Read the model definition and answer for the solid it produces. Units are mm, in the model's axes. A direction names the side the tool comes from. Give positions to 0.01 mm unless a question says otherwise; leave off trailing zeros. Loops run counter-clockwise (first coordinate to the right, second up) from the corner with the lowest first, then second, coordinate; pieces in that order, holes last. Notation, with made-up numbers: (35, -10) -> (66, -10) arc R30 ccw to (66, 13) -> close; hole circle Ø6 at (40, -6.75). An arc over 180 degrees is marked (long way). Return JSON: item names as keys, results as strings. Group by question number.
from build123d import *

# Parameters (mm, degrees)
SKETCH2_R           = 1.7
SKETCH2_R_2         = 2.5527
SKETCH2_R_3         = 1
SKETCH2_R_4         = 6.275
BOSS_EXTRUDE1_DEPTH = 5.588
FILLET1_R           = 6.35
FILLET2_R           = 3.175


with BuildPart() as part:
    # Sketch2 → Boss-Extrude1 (new body)
    with BuildSketch(Plane.XY):
        Polygon((-44.45, 12.7), (-101.6, 12.7), (-101.6, 6.35), (-107.95, 6.35), (-107.95, 3.175), (-101.6, 3.175), (-101.6, -3.175), (-107.95, -3.175), (-107.95, -6.35), (-101.6, -6.35), (-101.6, -12.7), (85.725, -12.7), (85.725, -20.9775), (92.075, -20.9775), (92.075, -12.7), (101.6, -12.7), (101.6, 12.7), (92.075, 12.7), (92.075, 20.9775), (85.725, 20.9775), (85.725, 12.7), (44.45, 12.7), (44.45, 15.875), (41.275, 15.875), (41.275, 12.7), (34.925, 12.7), (34.925, 15.875), (31.75, 15.875), (31.75, 12.7), (-31.75, 12.7), (-31.75, 15.875), (-34.925, 15.875), (-34.925, 12.7), (-41.275, 12.7), (-41.275, 15.875), (-44.45, 15.875), align=None)
        with BuildLine():
            ThreePointArc((-92.075, -3.175), (-95.25, 0), (-92.075, 3.175))
            Line((-92.075, 3.175), (-73.025, 3.175))
            ThreePointArc((-73.025, 3.175), (-69.85, 0), (-73.025, -3.175))
            Line((-73.025, -3.175), (-92.075, -3.175))
        make_face(mode=Mode.SUBTRACT)
        with Locations((-53.975, -9.525)):
            Circle(SKETCH2_R, mode=Mode.SUBTRACT)
        with Locations((-38.1, 0)):
            Circle(SKETCH2_R_2, mode=Mode.SUBTRACT)
        with Locations((-12.7, 0)):
            Circle(SKETCH2_R_2, mode=Mode.SUBTRACT)
        with Locations((88.9, -16.215)):
            Circle(SKETCH2_R_3, mode=Mode.SUBTRACT)
        with Locations((12.7, 0)):
            Circle(SKETCH2_R_2, mode=Mode.SUBTRACT)
        with Locations((38.1, 0)):
            Circle(SKETCH2_R_2, mode=Mode.SUBTRACT)
        with Locations((69.85, -9.525)):
            Circle(SKETCH2_R, mode=Mode.SUBTRACT)
        with Locations((88.9, 0)):
            Circle(SKETCH2_R_4, mode=Mode.SUBTRACT)
        with Locations((-53.975, 9.525)):
            Circle(SKETCH2_R, mode=Mode.SUBTRACT)
        with Locations((69.85, 9.525)):
            Circle(SKETCH2_R, mode=Mode.SUBTRACT)
        with Locations((88.9, 16.215)):
            Circle(SKETCH2_R_3, mode=Mode.SUBTRACT)
    extrude(amount=BOSS_EXTRUDE1_DEPTH)

    # Fillet1
    fillet1_edges = [part.edges().sort_by_distance(p)[0] for p in [
        (101.6, -12.7, 2.794),
        (101.6, 12.7, 2.794),
        (-101.6, -12.7, 2.794),
        (-101.6, 12.7, 2.794),
        (85.725, -12.7, 2.794),
        (85.725, 12.7, 2.794),
    ]]
    fillet(fillet1_edges, radius=FILLET1_R - 0.0001)  # a hair under: the kernel refuses the full size

    # Fillet2
    fillet2_edges = [part.edges().sort_by_distance(p)[0] for p in [
        (85.725, -20.9775, 2.794),
        (92.075, -20.9775, 2.794),
        (92.075, -12.7, 2.794),
        (92.075, 12.7, 2.794),
        (92.075, 20.9775, 2.794),
        (85.725, 20.9775, 2.794),
    ]]
    fillet(fillet2_edges, radius=FILLET2_R)


solid = part.part
1. Section B-B on z = 4.4 is taken. State how many separate pieces and enclosed holes the cut face has, then the cut area to 3 significant figures.
2. Straight lines are drawn through the part: line 1 (Y direction, x = 88.9, z = 3.7) (1 decimal); line 2 (Y direction, x = -77, z = 4.5) (3 decimals); line 3 (X direction, y = -8, z = 3.6). For each, find the intervals that lie inside material, in ascending order. Write a range as from..to.
3. Determine the mould class of faces 6 (the flat face through (-69, 12.7, 3)), 7 (the flat face through (-38, 12.7, 3)), 8 (the cylindrical face through (99.69, -10.89, 2.83)) for opening direction X: pulls with the +X half, pulls with the -X half, needs draft (parallel to the pull), parting line crosses it, or undercut.
4. Section A-A on x = -12.7 is taken. Determine the outline of the cut face in (y, z), then the cut area to 3 significant figures.
5. Which of the six approach directions +Z, -Z, +X, -X, +Y, -Y give full straight-line access (tool end or side, diameter ignored) to faces 1 (the flat face through (-105, -3.175, 3)), 2 (the flat face through (-9, -12.7, 3)), 3 (the flat face through (-105, 6.35, 3)), 4 (the flat face through (38, 12.7, 3)), 5 (the flat face through (-83, 3.175, 3))?
6. Flat-ended cylindrical pins translate along their axes: pin 1 Ø3 at (y, z) = (1, 3) entering from -X; pin 2 Ø3 at (x, z) = (-106, 1.5) entering from +Y; pin 3 Ø2.5 at (x, z) = (-43.5, 2.5) entering from +Y (3 decimals). Find the tip coordinate at first contact, or state that the pin passes through.
Completed:
{
 "1": {"separate pieces": "1", "enclosed holes": "12", "area": "4,930 mm²"},
 "2": {"line 1": "y = -21..-17.2, -15.2..-6.3, 6.3..15.2, 17.2..21", "line 2": "y = -12.7..-3.175, 3.175..12.7", "line 3": "x = -101.38..-54.73, -53.22..69.1, 70.6..101.38"},
 "3": {"face 6": "needs draft", "face 7": "undercut", "face 8": "pulls with the +X half"},
 "4": {"outline": "(-12.7, 0) -> (-2.55, 0) -> (-2.55, 5.59) -> (-12.7, 5.59) -> close; (2.55, 0) -> (12.7, 0) -> (12.7, 5.59) -> (2.55, 5.59) -> close", "area": "113 mm²"},
 "5": {"face 1": "+Z, -Z, -X", "face 2": "+Z, -Z, -X, -Y", "face 3": "+Z, -Z, -X, +Y", "face 4": "+Z, -Z, +Y", "face 5": "+Z, -Z"},
 "6": {"pin 1": "stops at x = -101.6", "pin 2": "stops at y = 6.35", "pin 3": "stops at y = 15.875"}
}
